The model under review builds one solid part; all positions refer to its coordinate system, in mm. A direction names the side the tool comes from. Round coordinates to 2 decimals unless told otherwise and drop trailing zeros. Loops run counter-clockwise (first coordinate to the right, second up) from the corner with the lowest first, then second, coordinate; pieces in that order, holes last. Notation, with made-up numbers: M 3,42 L 9,42 A17 cw 9,62 Z; hole C 81,-2.75 d11. An arc over 180 degrees is marked long. Answer as a JSON object with one key per item and string values. Group by question number.
Item 1: Consider section C-C (y = 7). Give the boundary of the cut face in (x, z).
Item 2: Consider section A-A (x = 7). Give the boundary of the cut face in (y, z).
Item 3: Insertion check: P1, Ø0.9, axis at x = 2.5, z = -2.5, coming from the -Y side; P2, Ø1.5, axis at y = 4, z = 2.5, coming from the +X side; P3, Ø1, axis at y = 4, z = 0.5, coming from the -X side. Each pin has a flat end and moves straight along its axis. Give the tip position at first contact, or say it passes through.
Item 4: Tool access review of faces 4 (the face through (9.55, 0.43, 3.02)), 5 (the face through (0, 0, 3)), 6 (the face through (3.653, 9.872, 4.007)): name each direction out of +Z, -Z, +X, -X, +Y, -Y from which nothing blocks a thin tool from reaching the whole face with its end or side.
Item 5: To check wall thickness, follow line 1 (X direction, y = 5.75, z = 4); line 2 (X direction, y = 9.25, z = 0); line 3 (Z direction, x = 4.25, y = 4). State the ranges of each line that lie inside material, in increasing order.
Item 6: The part is to be moulded in two halves that separate along Y. For faces 1 (the face through (-1, 11, 4.5)), 2 (the face through (-1, 6.306, 4)), 3 (the face through (0, 20, 3)), say which applies: +Y half, -Y half, draft (parallel to the pull), parting line (faces both ways), or undercut.
Item 7: Consider section D-D (y = 4). Give the boundary of the cut face in (x, z), and give its area (3 significant figures).
Item 8: Consider section B-B (z = -2.75). Give the boundary of the cut face in (x, y), and give its area (3 significant figures).
```python
from build123d import *

# Parameters (mm, degrees)
F0_W     = 14
F0_H     = 3
F0_W_2   = 3
F1_DEPTH = 20
F2_DEPTH = 3
F3_W     = 3
F3_H     = 3
F4_DEPTH = 100
F5_W     = 3
F5_H     = 3.5
F6_DEPTH = 100
F7_R     = 1.5
F9_DEPTH = 1


with BuildPart() as f1:
    # F0 (on Front) → F1 (new body)
    with BuildSketch(Plane.XZ):
        Polygon((10, 1.5), (10, 4.5), (-10, 4.5), (-10, 1.5), (-7, 1.5), (7, 1.5), align=None)
        Rectangle(F0_W, F0_H)
        with Locations((11.5, 0)):
            Rectangle(F0_W_2, F0_H)
        with Locations((8.5, 0)):
            Rectangle(F0_W_2, F0_H)
        with Locations((-8.5, 0)):
            Rectangle(F0_W_2, F0_H)
        Polygon((10, -4.5), (10, -1.5), (7, -1.5), (-7, -1.5), (-10, -1.5), (-10, -4.5), align=None)
    extrude(amount=-F1_DEPTH)

    # F0 (on Front) → F2 (join)
    with BuildSketch(Plane.XZ):
        with Locations((-8.5, 0)):
            Rectangle(F0_W_2, F0_H)
        Rectangle(F0_W, F0_H)
        with Locations((8.5, 0)):
            Rectangle(F0_W_2, F0_H)
        with Locations((11.5, 0)):
            Rectangle(F0_W_2, F0_H)
    extrude(amount=F2_DEPTH)

    # F3 (on face) → F4 (cut)
    with BuildSketch(Plane.YZ.offset(13)):
        Polygon((23, -1.75), (23, 1.75), (17, 1.75), (17, 1.5), (20, 1.5), (20, -1.5), (17, -1.5), (17, -1.75), align=None)
        with Locations((18.5, 0)):
            Rectangle(F3_W, F3_H)
    extrude(amount=-F4_DEPTH, mode=Mode.SUBTRACT)

    # F5 (on face) → F6 (cut)
    with BuildSketch(Plane(origin=(0, 17, 0), x_dir=(-1, 0, 0), z_dir=(0, 1, 0))):
        with Locations((11.5, 0)):
            Rectangle(F5_W, F5_H)
        with Locations((8.5, 0)):
            Rectangle(F5_W, F5_H)
    extrude(amount=-F6_DEPTH, mode=Mode.SUBTRACT)

    # F7
    f7_edges = [f1.edges().sort_by_distance(p)[0] for p in [
        (-7, -3, 0),
        (13, -3, 0),
        (10, 0, 3),
        (10, 0, -3),
        (-10, 0, -3.125),
        (-10, 0, 3.125),
        (-7, 17, 0),
        (-10, 20, 3.125),
        (-10, 20, -3.125),
        (13, 17, 0),
        (10, 20, 3.125),
        (10, 20, -3.125),
    ]]
    fillet(f7_edges, radius=F7_R)

    # F8 (on face) → F9 (cut)
    with BuildSketch(Plane.XY.offset(4.5)):
        with BuildLine():
            Line((0, 12.6293993567), (0, 16.9392361111))
            Line((0, 16.9392361111), (-2.4381510417, 16.9392361111))
            Line((-2.4381510417, 16.9392361111), (-7.3387586806, 3))
            Line((-7.3387586806, 3), (-4.1668836806, 3))
            Line((-4.1668836806, 3), (-3.1612413194, 6.3055555556))
            Line((-3.1612413194, 6.3055555556), (0, 6.3055555556))
            Line((0, 6.3055555556), (0, 8.7725694444))
            Line((0, 8.7725694444), (-2.419921875, 8.7725694444))
            add(Edge.make_bspline(
                [(-0.6273871528, 14.7821180556), (-0.9403211806, 13.5668402778), (-2.419921875, 8.7725694444)],
                knots=[0, 0, 0, 1, 1, 1], degree=2))
            add(Edge.make_bspline(
                [(-0.3752170139, 13.8524305556), (-0.5514322917, 14.4418402778), (-0.6273871528, 14.7821180556)],
                knots=[0, 0, 0, 1, 1, 1], degree=2))
            add(Edge.make_bspline(
                [(0, 12.6293993567), (-0.2996453455, 13.5996563543), (-0.3752170139, 13.8524305556)],
                knots=[0.5711400886, 0.5711400886, 0.5711400886, 1, 1, 1], degree=2))
        make_face()
        with BuildLine():
            Line((1.1590711806, 16.9392361111), (0, 16.9392361111))
            Line((0, 16.9392361111), (0, 12.6293993567))
            add(Edge.make_bspline(
                [(1.1955295139, 8.7725694444), (0.3990568122, 11.3372462484), (0, 12.6293993567)],
                knots=[0, 0, 0, 0.5711400886, 0.5711400886, 0.5711400886], degree=2))
            Line((1.1955295139, 8.7725694444), (0, 8.7725694444))
            Line((0, 8.7725694444), (0, 6.3055555556))
            Line((0, 6.3055555556), (1.900390625, 6.3055555556))
            Line((1.900390625, 6.3055555556), (2.9060329861, 3))
            Line((2.9060329861, 3), (6.0779079861, 3))
            Line((6.0779079861, 3), (1.1590711806, 16.9392361111))
        make_face()
    extrude(amount=-F9_DEPTH, mode=Mode.SUBTRACT)


solid = f1.part
```
Geometry results:
{
 "1": {"outline": "M -10,-4.5 L 10,-4.5 L 10,-1.5 L 13,-1.5 L 13,1.5 L 10,1.5 L 10,4.5 L 4.67,4.5 L 4.67,3.5 L -5.93,3.5 L -5.93,4.5 L -10,4.5 L -10,1.75 L -7,1.75 L -7,-1.75 L -10,-1.75 Z"},
 "2": {"outline": "M -3,-1.5 L 0,-1.5 L 0,-4.5 L 20,-4.5 L 20,-1.75 L 17,-1.75 L 17,1.75 L 20,1.75 L 20,4.5 L 0,4.5 L 0,1.5 L -3,1.5 Z"},
 "3": {"P1": "stops at y = 0", "P2": "stops at x = 10", "P3": "stops at x = -7"},
 "4": {"face 4": "+Z, +X, -Y", "face 5": "+Z, +X, -X, -Y", "face 6": "+Z"},
 "5": {"line 1": "x = -10 to -6.37, -3.33 to 2.07, 5.11 to 10", "line 2": "x = -7 to 13", "line 3": "z = -4.5 to 3.5"},
 "6": {"face 1": "draft", "face 2": "undercut", "face 3": "+Y half"},
 "7": {"outline": "M -10,-4.5 L 10,-4.5 L 10,-1.5 L 13,-1.5 L 13,1.5 L 10,1.5 L 10,4.5 L 5.73,4.5 L 5.73,3.5 L 2.6,3.5 L 2.6,4.5 L -3.86,4.5 L -3.86,3.5 L -6.99,3.5 L -6.99,4.5 L -10,4.5 L -10,1.75 L -7,1.75 L -7,-1.75 L -10,-1.75 Z", "area": "172 mm^2"},
 "8": {"outline": "M -10,1.5 A1.5 ccw -8.5,0 L 8.5,0 A1.5 ccw 10,1.5 L 10,18.5 A1.5 ccw 8.5,20 L -8.5,20 A1.5 ccw -10,18.5 Z", "area": "398 mm^2"}
}
